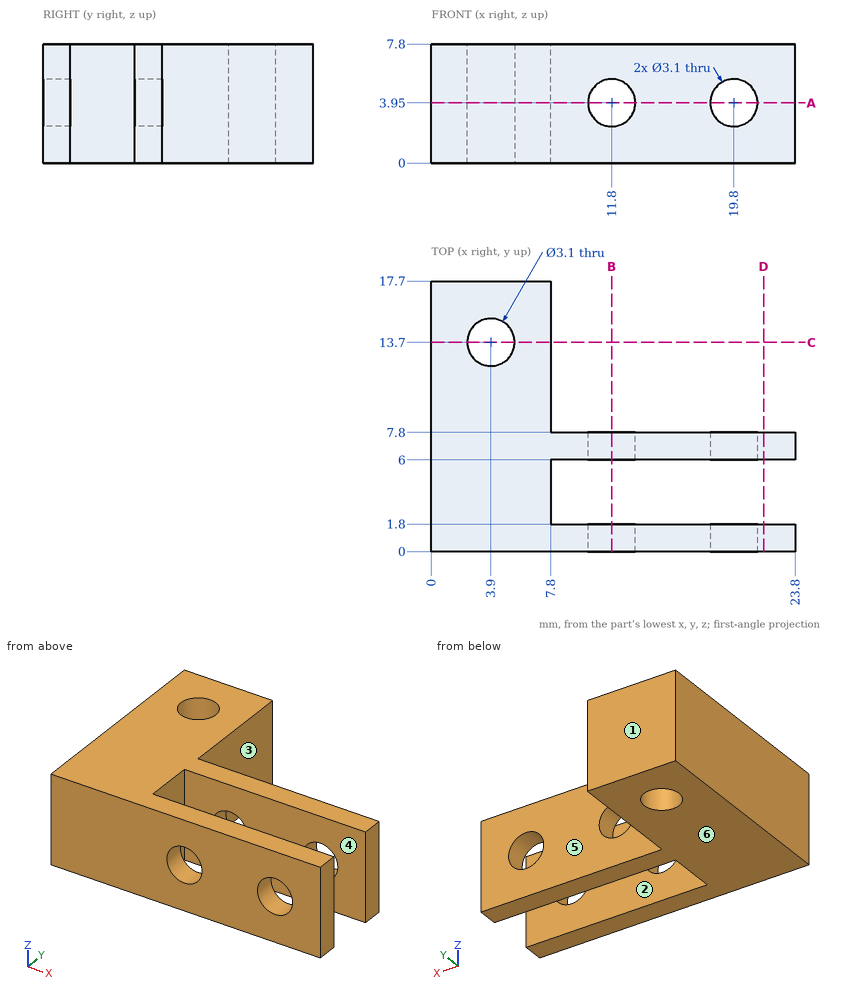
Source: three-view drawing plus pictorial views. Frame: mm from the lowest corner of the part. A direction names the side the tool comes from. Round coordinates to 2 decimals unless told otherwise and drop trailing zeros. Order: outer loops, then holes, each group sorted by start corner. A loop starts at its lowest first (then second) coordinate and runs counter-clockwise, first axis right, second up. Notation, with made-up numbers: (-4, -24) -> (24, -24) arc R24 ccw to (24, -11) -> close; hole circle Ø3 at (7, 65). An arc over 180 degrees is marked (long way). Use CSV: the item, a comma, the result in double quotes. Start each with the question number.
1) Draft query along Y for the marked faces 4, 5 and 6. Return one class per face: +Y half, -Y half, draft (parallel to the pull), parting line (faces both ways), or undercut.
2) Section D-D (x = 21.75). Return the cut outline in (y, z).
3) First-contact query: pin 1 Ø1 at (x, y) = (8.5, 14) entering from -Z; pin 2 Ø1.5 at (x, z) = (8.5, 3) entering from +Y; pin 3 Ø2.5 at (x, z) = (19.5, 5) entering from +Y; pin 4 Ø1 at (y, z) = (10, 3) entering from +X. Flat tips, straight axial feed; report the tip coordinate or a pass-through.
4) Set-up query: the marked faces 1, 2 and 3. Return all of +Z, -Z, +X, -X, +Y, -Y with unobstructed straight access to the full face (end or side cutting, diameter ignored); none if empty.
5) Section A-A (z = 3.95). Return the cut outline in (x, y).
6) Section B-B (x = 11.8). Return the cut outline in (y, z).
7) Material intervals for line 1 along Z through (x, y) = (11.8, 0.9); line 2 along Y through (x, z) = (3.9, 2.5); line 3 along Y through (x, z) = (17.5, 5.5), sorted ascending. Write a range as from..to.
8) Section C-C (y = 13.7). Return the cut outline in (x, z), and give its area (3 significant figures).
Returned:
1,face 4,"undercut"
1,face 5,"+Y half"
1,face 6,"draft"
2,outline,"(0, 0) -> (1.8, 0) -> (1.8, 7.8) -> (0, 7.8) -> close; (6, 0) -> (7.8, 0) -> (7.8, 7.8) -> (6, 7.8) -> close"
3,pin 1,"passes through"
3,pin 2,"stops at y = 17.7"
3,pin 3,"stops at y = 7.8"
3,pin 4,"stops at x = 7.8"
4,face 1,"+Z, -Z, +X, -X, +Y"
4,face 2,"+Z, -Z, +X"
4,face 3,"+Z, -Z, +X, +Y"
5,outline,"(0, 0) -> (10.25, 0) -> (10.25, 1.8) -> (7.8, 1.8) -> (7.8, 6) -> (10.25, 6) -> (10.25, 7.8) -> (7.8, 7.8) -> (7.8, 17.7) -> (0, 17.7) -> close; (13.35, 0) -> (18.25, 0) -> (18.25, 1.8) -> (13.35, 1.8) -> close; (13.35, 6) -> (18.25, 6) -> (18.25, 7.8) -> (13.35, 7.8) -> close; (21.35, 0) -> (23.8, 0) -> (23.8, 1.8) -> (21.35, 1.8) -> close; (21.35, 6) -> (23.8, 6) -> (23.8, 7.8) -> (21.35, 7.8) -> close; hole circle Ø3.1 at (3.9, 13.7)"
6,outline,"(0, 0) -> (1.8, 0) -> (1.8, 2.4) -> (0, 2.4) -> close; (0, 5.5) -> (1.8, 5.5) -> (1.8, 7.8) -> (0, 7.8) -> close; (6, 0) -> (7.8, 0) -> (7.8, 2.4) -> (6, 2.4) -> close; (6, 5.5) -> (7.8, 5.5) -> (7.8, 7.8) -> (6, 7.8) -> close"
7,line 1,"z = 0..2.4, 5.5..7.8"
7,line 2,"y = 0..12.15, 15.25..17.7"
7,line 3,"y = 0..1.8, 6..7.8"
8,outline,"(0, 0) -> (2.35, 0) -> (2.35, 7.8) -> (0, 7.8) -> close; (5.45, 0) -> (7.8, 0) -> (7.8, 7.8) -> (5.45, 7.8) -> close"
8,area,"36.7 mm²"
